Could you check a few things on this model? Use its own coordinates, in mm. A direction names the side the tool comes from. Give positions to 0.01 mm unless a question says otherwise; leave off trailing zeros. Loops run counter-clockwise (first coordinate to the right, second up) from the corner with the lowest first, then second, coordinate; pieces in that order, holes last.
1. For faces 1 (the flat face through (-23.5, 2, 0)), 2 (the flat face through (12.5, 0.7, -10.7)), 3 (the flat face through (-22.5, 3, 0)), which set-ups out of +Z, -Z, +X, -X, +Y, -Y let a thin tool reach every point of the face, with its end or its side?
2. Imagine slicing it at A-A (z = -5.5). List the corners of the cut face in (x, y) for me, plus the area to 3 significant figures.
3. Imagine slicing it at D-D (z = 19.5). List the corners of the cut face in (x, y) for me, plus the area to 3 significant figures.
4. I need wall thicknesses on line 1 along X through (y, z) = (3.3, -7); line 2 along X through (y, z) = (0.9, -16). Which ranges of each line are inside material? Lowest first, please.
5. Imagine slicing it at C-C (x = -19.5). List the corners of the cut face in (y, z) for me.
6. For P1, Ø3.5, axis at x = 20, z = -19, coming from the +Y side; P2, Ø4, axis at x = 8.5, z = 16.5, coming from the -Y side; P3, Ø0.8, axis at x = 1, y = 0.5, coming from the -Z side; P4, Ø22.5, axis at x = -8, z = -6.5, coming from the +Y side, each with a flat end and sliding along its axis, tell me the tip position at first contact or that it passes through.
7. Imagine slicing it at B-B (y = 3.6). List the corners of the cut face in (x, z) for me.
8. Thinking about a two-plate mould opening in Z: for faces 4 (the flat face through (-0.2, 0.5, 6.5)), 5 (the flat face through (0, 2, 23.5)), 6 (the flat face through (-12.5, 0.7, -10.8)), 7 (the flat face through (18, 3, -22.5)), which applies, +Z half, -Z half, draft (parallel to the pull), parting line (faces both ways), or undercut?
Autodesk Inventor part; units mm, degrees
ref_plane "YZ Plane" through (0, 0, 0) normal (1, 0, 0) x (0, 1, 0)
ref_plane "XZ Plane" through (0, 0, 0) normal (0, 1, 0) x (-1, 0, 0)
ref_plane "XY Plane" through (0, 0, 0) normal (0, 0, 1) x (1, 0, 0)
sketch "Sketch1" plane through (0, 0, 0) normal (0, 1, 0) x (-1, 0, 0)
  point P0 (0, 0)
sketch "Sketch2" plane through (0, 0, 0) normal (0, 1, 0) x (-1, 0, 0)
  line L0 (23.5, 23.5) -> (-23.5, 23.5)
  line L1 (-23.5, 23.5) -> (-23.5, -23.5)
  line L2 (-23.5, -23.5) -> (23.5, -23.5)
  line L3 (23.5, -23.5) -> (23.5, 23.5)
  point P0 (0, 0)
  dimension "d4" = 47
  dimension "d5" = 47
  dimension "d6" = 23.5
  dimension "d7" = 23.5
extrude "Extrusion1" add sketch "Sketch2" along normal blind 5
sketch "Sketch3" plane through (0, 5, 0) normal (0, 1, 0) x (1, 0, 0)
  point P0 (0, 0)
sketch "Sketch4" plane through (0, 5, 0) normal (0, 1, 0) x (1, 0, 0)
  line L0 (-22.5, -22.5) -> (22.5, -22.5)
  line L1 (22.5, -22.5) -> (22.5, 22.5)
  line L2 (22.5, 22.5) -> (-22.5, 22.5)
  line L3 (-22.5, 22.5) -> (-22.5, -22.5)
  point P0 (0, 0)
  dimension "d10" = 45
  dimension "d11" = 45
  dimension "d12" = 22.5
  dimension "d13" = 22.5
extrude "Extrusion2" cut sketch "Sketch4" against normal blind 4
sketch "Sketch5" plane through (0, 5, 0) normal (0, 1, 0) x (1, 0, 0)
  line L0 (23.5, 23.5) -> (-23.5, 23.5)
  line L1 (12.5, 23.5) -> (-12.5, 23.5)
  line L2 (-12.5, 23.5) -> (-12.5, -6.5)
  line L3 (-12.5, -6.5) -> (12.5, -6.5)
  line L4 (12.5, -6.5) -> (12.5, 23.5)
  point P0 (0, 0)
  dimension "d16" = 30
  dimension "d17" = 25
  dimension "d18" = 12.5
extrude "Extrusion3" cut sketch "Sketch5" against normal blind 10
sketch "Sketch6" plane through (0, 1, 0) normal (0, 1, 0) x (1, 0, 0)
  circle A0 centre (-19.5, -19.5) radius 1.5
  line L0 (-23.5, 23.5) -> (-23.5, -23.5)
  line L1 (-23.5, -23.5) -> (23.5, -23.5)
  line L2 (0, 0) -> (-11.992, 0) construction
  line L3 (0, 0) -> (0, -9.7427) construction
  circle A1 centre (-19.5, 19.5) radius 1.5
  line L4 (-22.5, -22.5) -> (-22.5, 22.5)
  line L5 (22.5, -22.5) -> (-22.5, -22.5)
  circle A2 centre (19.5, -19.5) radius 1.5
  circle A3 centre (19.5, 19.5) radius 1.5
  dimension "d21" = 3
  dimension "d24" = 3
  dimension "d25" = 3
  dimension "d26" = 3
  dimension "d27" = 3
  dimension "d28" = 3
extrude "Extrusion4" add sketch "Sketch6" along normal blind 1
properties part number "particle_sensor_case_bottom"
Derived:
1. face 1: +Z, -Z, -X, +Y, -Y
1. face 2: -Z, +Y, -Y
1. face 3: +Y
2. outline: (-23.5, 0) - (-12.5, 0) - (-12.5, 1) - (-22.5, 1) - (-22.5, 5) - (-23.5, 5) - close; (12.5, 0) - (23.5, 0) - (23.5, 5) - (22.5, 5) - (22.5, 1) - (12.5, 1) - close
2. area: 30.0 mm2
3. outline: (-23.5, 0) - (23.5, 0) - (23.5, 5) - (22.5, 5) - (22.5, 1) - (21, 1) - (21, 2) - (18, 2) - (18, 1) - (-18, 1) - (-18, 2) - (-21, 2) - (-21, 1) - (-22.5, 1) - (-22.5, 5) - (-23.5, 5) - close
3. area: 61.0 mm2
4. line 1: x = -23.5 to -22.5, 22.5 to 23.5
4. line 2: x = -23.5 to -12.5, 12.5 to 23.5
5. outline: (0, -23.5) - (5, -23.5) - (5, -22.5) - (1, -22.5) - (1, -21) - (2, -21) - (2, -18) - (1, -18) - (1, 18) - (2, 18) - (2, 21) - (1, 21) - (1, 22.5) - (5, 22.5) - (5, 23.5) - (0, 23.5) - close
6. P1: stops at y = 2
6. P2: stops at y = 0
6. P3: stops at z = 6.5
6. P4: stops at y = 1
7. outline: (-23.5, -23.5) - (-12.5, -23.5) - (-12.5, -22.5) - (-22.5, -22.5) - (-22.5, 22.5) - (22.5, 22.5) - (22.5, -22.5) - (12.5, -22.5) - (12.5, -23.5) - (23.5, -23.5) - (23.5, 23.5) - (-23.5, 23.5) - close
8. face 4: -Z half
8. face 5: +Z half
8. face 6: draft
8. face 7: undercut
